Job drawing, mm, ordinate dimensions from the low corner. One solid piece. A direction names the side the tool comes from. Round coordinates to 2 decimals unless told otherwise and drop trailing zeros. Order: outer loops, then holes, each group sorted by start corner. A loop starts at its lowest first (then second) coordinate and runs counter-clockwise, first axis right, second up. Notation, with made-up numbers: (-28, -40) -> (19, -40) arc R23 cw to (19, -29) -> close; hole circle Ø10 at (25, -26.75). An arc over 180 degrees is marked (long way). Return JSON: item names as keys, results as strings. Group by question number.
Q1. Cut at A-A (x = 12). Write the cut outline in (y, z).
Q2. Probe line 1 along Z through (x, y) = (9, 26); line 2 along Y through (x, z) = (20, 29). List the from-to ranges inside material, lowest first.
Q3. Cut at B-B (y = 22). Write the cut outline in (x, z), then the cut area to 3 significant figures.
Q4. Flat gauge pin, fed straight in: pin 1 (9.5 mm diameter, centred on x = 29, y = 9.5, fed in from +Z). Where does the tip first touch, or does it go through?
Q5. Which spindle directions (+Z, -Z, +X, -X, +Y, -Y) get a long thin tool onto all of the face, cutting with end or side? Do the marked faces 1 and 2. Say none if no direction does.
Q6. Cut at C-C (z = 28). Write the cut outline in (x, y).
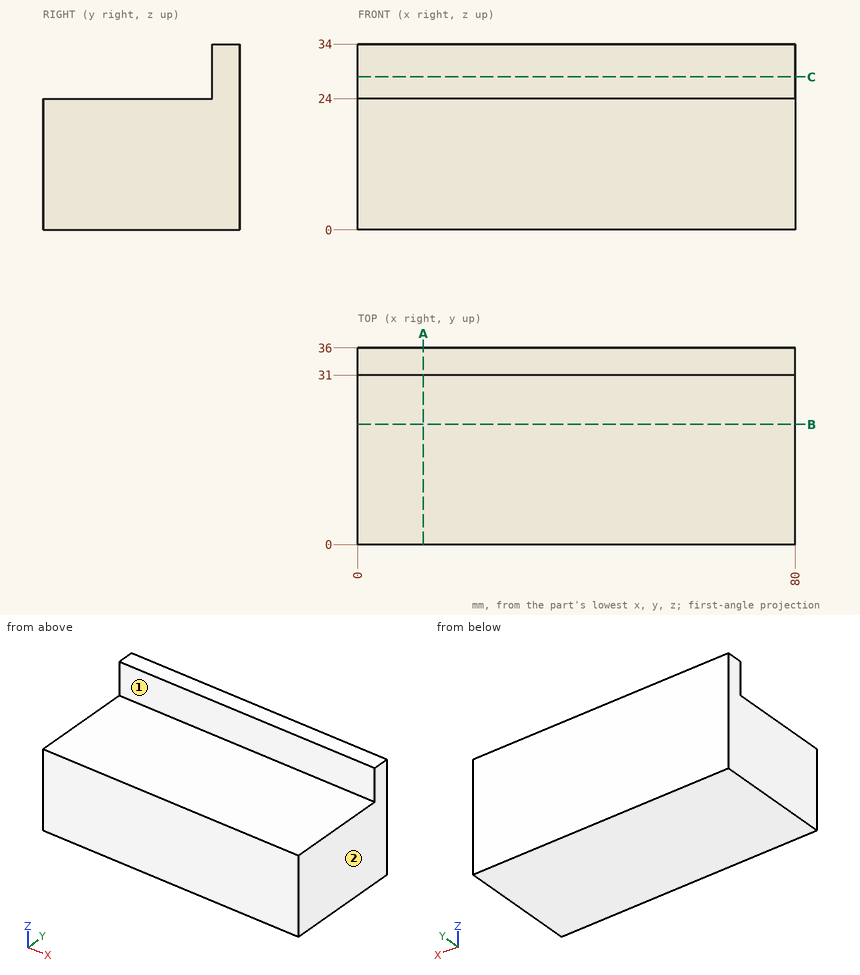
Solution:
{
 "1": {"outline": "(0, 0) -> (36, 0) -> (36, 34) -> (31, 34) -> (31, 24) -> (0, 24) -> close"},
 "2": {"line 1": "z = 0 to 24", "line 2": "y = 31 to 36"},
 "3": {"outline": "(0, 0) -> (80, 0) -> (80, 24) -> (0, 24) -> close", "area": "1,920 mm²"},
 "4": {"pin 1": "stops at z = 24"},
 "5": {"face 1": "+Z, +X, -X, -Y", "face 2": "+Z, -Z, +X, +Y, -Y"},
 "6": {"outline": "(0, 31) -> (80, 31) -> (80, 36) -> (0, 36) -> close"}
}
